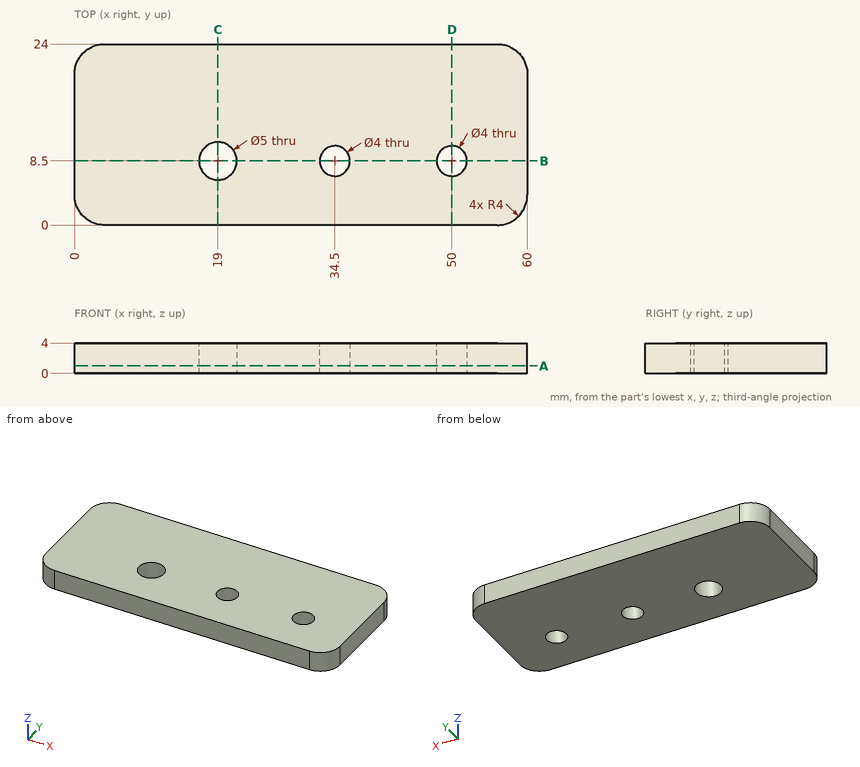
Design review of the part shown in the three views and the two pictorial views. Dimensions are in mm from the part's minimum x, y and z. Round coordinates to 2 decimals unless told otherwise and drop trailing zeros. Write each loop counter-clockwise with the first axis right and the second up, starting at its lowest first coordinate (ties: lowest second). Pieces come first, ordered by that corner, then holes.
Item 1: We need section B-B on y = 8.5. Write out the cut boundary in (x, z).
Item 2: We need section A-A on z = 1. Write out the cut boundary in (x, y).
Item 3: We need section C-C on x = 19. Write out the cut boundary in (y, z), and give its area (3 significant figures).
Item 4: For probe 1 along Y at (x, z) = (19, 2.65); probe 2 along Y at (x, z) = (34.5, 1.45); probe 3 along X at (y, z) = (8, 1.25), list the stretches that pass through material, from the lowest coordinate up.
Item 5: Clearance check with a flat-ended pin moving along its axis: pin 1 Ø2 at (x, z) = (18, 1) entering from -Y. State where the tip first meets the part, or that it passes through.
Item 6: We need section D-D on x = 50. Write out the cut boundary in (y, z), and give its area (3 significant figures).
Returned:
1. outline: (0, 0) - (16.5, 0) - (16.5, 4) - (0, 4) - close; (21.5, 0) - (32.5, 0) - (32.5, 4) - (21.5, 4) - close; (36.5, 0) - (48, 0) - (48, 4) - (36.5, 4) - close; (52, 0) - (60, 0) - (60, 4) - (52, 4) - close
2. outline: (0, 4) arc R4 ccw to (4, 0) - (56, 0) arc R4 ccw to (60, 4) - (60, 20) arc R4 ccw to (56, 24) - (4, 24) arc R4 ccw to (0, 20) - close; hole circle Ø5 at (19, 8.5); hole circle Ø4 at (34.5, 8.5); hole circle Ø4 at (50, 8.5)
3. outline: (0, 0) - (6, 0) - (6, 4) - (0, 4) - close; (11, 0) - (24, 0) - (24, 4) - (11, 4) - close
3. area: 76.0 mm2
4. probe 1: y = 0 to 6, 11 to 24
4. probe 2: y = 0 to 6.5, 10.5 to 24
4. probe 3: x = 0 to 16.55, 21.45 to 32.56, 36.44 to 48.06, 51.94 to 60
5. pin 1: stops at y = 0
6. outline: (0, 0) - (6.5, 0) - (6.5, 4) - (0, 4) - close; (10.5, 0) - (24, 0) - (24, 4) - (10.5, 4) - close
6. area: 80.0 mm2
